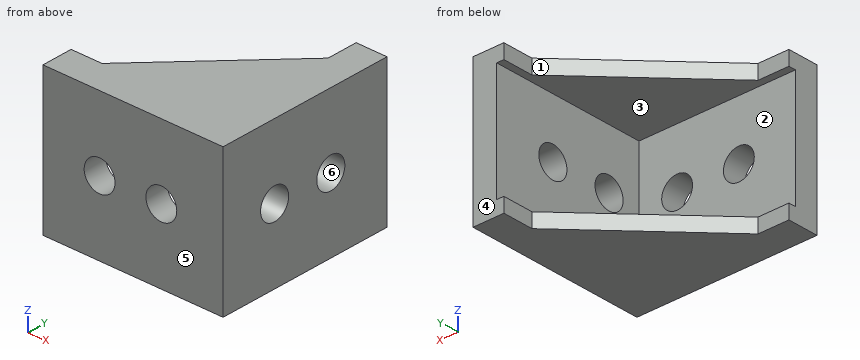
```python
from build123d import *

# Parameters (mm, degrees)
EXTRUDE_1_DEPTH     = 14.15
SKETCH_2_W          = 30.4
SKETCH_2_H          = 30.4
CUT_EXTRUDE_1_DEPTH = 11.35
CUT_EXTRUDE_2_REACH = 53.48
SKETCH_4_R          = 3
CUT_EXTRUDE_3_REACH = 53.48
SKETCH_5_R          = 3


with BuildPart() as part:
    # 草图1 → 凸台-拉伸1 (new, symmetric)
    with BuildSketch(Plane.XY):
        Polygon((0, 0), (35, 0), (35, 35), (29, 35), (29, 29), (6, 6), (0, 6), align=None)
    extrude(amount=EXTRUDE_1_DEPTH, both=True)

    # 草图2 → 切除-拉伸1 (cut, symmetric)
    with BuildSketch(Plane.XY):
        with Locations((15.2, 19.8)):
            Rectangle(SKETCH_2_W, SKETCH_2_H)
    extrude(amount=CUT_EXTRUDE_1_DEPTH, both=True, mode=Mode.SUBTRACT)

    # 草图4 → 切除-拉伸2 (cut, up to next)
    with BuildSketch(Plane(origin=(0, 0, 0), x_dir=(1, 0, 0), z_dir=(0, 1, 0)), mode=Mode.PRIVATE) as cut_extrude_2_sk1:
        with Locations(Location((23, 0, 0), (0, 0, 270))):
            Circle(SKETCH_4_R)
    cut_extrude_2_tool1 = extrude(cut_extrude_2_sk1.sketch, amount=CUT_EXTRUDE_2_REACH, mode=Mode.PRIVATE) & part.part
    # 草图4 → 切除-拉伸2 (cut, up to next)
    with BuildSketch(Plane(origin=(0, 0, 0), x_dir=(1, 0, 0), z_dir=(0, 1, 0)), mode=Mode.PRIVATE) as cut_extrude_2_sk2:
        with Locations(Location((11, 0, 0), (0, 0, 270))):
            Circle(SKETCH_4_R)
    cut_extrude_2_tool2 = extrude(cut_extrude_2_sk2.sketch, amount=CUT_EXTRUDE_2_REACH, mode=Mode.PRIVATE) & part.part
    add(cut_extrude_2_tool1.solids().sort_by_distance((23, 0, 0))[0], mode=Mode.SUBTRACT)
    add(cut_extrude_2_tool2.solids().sort_by_distance((11, 0, 0))[0], mode=Mode.SUBTRACT)

    # 草图5 → 切除-拉伸3 (cut, up to next)
    with BuildSketch(Plane(origin=(0, 0, 0), x_dir=(0, 0, -1), z_dir=(1, 0, 0)), mode=Mode.PRIVATE) as cut_extrude_3_sk1:
        with Locations(Location((0, 23, 0), (0, 0, 180))):
            Circle(SKETCH_5_R)
    cut_extrude_3_tool1 = extrude(cut_extrude_3_sk1.sketch, amount=CUT_EXTRUDE_3_REACH, mode=Mode.PRIVATE) & part.part
    # 草图5 → 切除-拉伸3 (cut, up to next)
    with BuildSketch(Plane(origin=(0, 0, 0), x_dir=(0, 0, -1), z_dir=(1, 0, 0)), mode=Mode.PRIVATE) as cut_extrude_3_sk2:
        with Locations(Location((0, 11, 0), (0, 0, 180))):
            Circle(SKETCH_5_R)
    cut_extrude_3_tool2 = extrude(cut_extrude_3_sk2.sketch, amount=CUT_EXTRUDE_3_REACH, mode=Mode.PRIVATE) & part.part
    add(cut_extrude_3_tool1.solids().sort_by_distance((0, 23, 0))[0], mode=Mode.SUBTRACT)
    add(cut_extrude_3_tool2.solids().sort_by_distance((0, 11, 0))[0], mode=Mode.SUBTRACT)


solid = part.part
```
The listing builds one solid part. Answer for the finished solid, in the listing's coordinates (mm). Face numbers are marked on the shaded views. A direction names the side the tool comes from. Round coordinates to 2 decimals unless told otherwise and drop trailing zeros. Loops run counter-clockwise (first coordinate to the right, second up) from the corner with the lowest first, then second, coordinate; pieces in that order, holes last.
Q1. Given pin 1 Ø3.5 at (x, z) = (11, 0) entering from +Y; pin 2 Ø1.5 at (y, z) = (11, -7.5) entering from -X; pin 3 Ø3 at (x, z) = (3.5, 12.5) entering from +Y; pin 4 Ø2 at (y, z) = (33.5, 13.5) entering from -X, each flat-ended and moving along its own axis, determine where each tip first touches the part or whether it passes through.
Q2. Section A-A, the plane y = 23 is taken. Determine the outline of the cut face in (x, z), then the cut area to 3 significant figures.
Q3. Which of the six approach directions +Z, -Z, +X, -X, +Y, -Y give full straight-line access (tool end or side, diameter ignored) to the marked faces 1 and 2?
Q4. Section B-B, the plane x = 11 is taken. Determine the outline of the cut face in (y, z).
Q5. Section D-D, the plane x = 18 is taken. Determine the outline of the cut face in (y, z).
Q6. For a pull along Y with two mould halves and no side action, classify the marked faces 3, 4, 5 and 6 as released by +Y, released by -Y, zero draft, split by the parting line, or undercut.
Q7. Section C-C, the plane z = 0 is taken. Determine the outline of the cut face in (x, y), then the cut area to 3 significant figures.
Q8. Find the intervals of material crossed by line 1 (X direction, y = 3.45, z = 0); line 2 (Z direction, x = 21.5, y = 9), in increasing order.
Completed:
1. pin 1: passes through
1. pin 2: stops at x = 30.4
1. pin 3: stops at y = 6
1. pin 4: stops at x = 29
2. outline: (23, -14.15) - (35, -14.15) - (35, -3) - (30.4, -3) - (30.4, -11.35) - (23, -11.35) - close; (23, 11.35) - (30.4, 11.35) - (30.4, 3) - (35, 3) - (35, 14.15) - (23, 14.15) - close
2. area: 144 mm2
3. face 1: +Z, -Z, -X, +Y
3. face 2: -X, +Y
4. outline: (0, -14.15) - (11, -14.15) - (11, -11.35) - (4.6, -11.35) - (4.6, -3) - (0, -3) - close; (0, 3) - (4.6, 3) - (4.6, 11.35) - (11, 11.35) - (11, 14.15) - (0, 14.15) - close
5. outline: (0, -14.15) - (18, -14.15) - (18, -11.35) - (4.6, -11.35) - (4.6, 11.35) - (18, 11.35) - (18, 14.15) - (0, 14.15) - close
6. face 3: zero draft
6. face 4: released by +Y
6. face 5: released by -Y
6. face 6: undercut
7. outline: (0, 0) - (8, 0) - (8, 4.6) - (0, 4.6) - close; (14, 0) - (20, 0) - (20, 4.6) - (14, 4.6) - close; (26, 0) - (35, 0) - (35, 8) - (30.4, 8) - (30.4, 4.6) - (26, 4.6) - close; (30.4, 14) - (35, 14) - (35, 20) - (30.4, 20) - close; (30.4, 26) - (35, 26) - (35, 35) - (30.4, 35) - close
7. area: 190 mm2
8. line 1: x = 0 to 8, 14 to 20, 26 to 35
8. line 2: z = -14.15 to -11.35, 11.35 to 14.15
